Job drawing, mm, ordinate dimensions from the low corner. One solid piece. A direction names the side the tool comes from. Coordinates: 2 decimals unless noted, no trailing zeros. Loops run counter-clockwise (first coordinate to the right, second up) from the corner with the lowest first, then second, coordinate; pieces in that order, holes last. Notation, with made-up numbers: M 31.25,20 L 88.25,20 A22 cw 88.25,48 Z; hole C 43.5,62.25 d1. An arc over 180 degrees is marked long. Answer as a JSON object with one key per item and string values. Group by question number.
1. Drop flat-ended pins along their axis: pin 1 Ø2.5 at (x, z) = (6.5, 5.5) entering from +Y; pin 2 Ø0.7 at (x, z) = (6.5, 5.5) entering from -Y; pin 3 Ø2 at (y, z) = (10.5, 2) entering from +X. Give the stop position or say it passes through.
2. Saw through at D-D on z = 4.25. Write the cut outline in (x, y).
3. Saw through at B-B on z = 7.25. Write the cut outline in (x, y).
4. Saw through at C-C on x = 5.75. Write the cut outline in (y, z).
5. Drill centre lines: L1, parallel to Y at x = 4, z = 3; L2, parallel to Y at x = 6.5, z = 5.75; L3, parallel to X at y = 9, z = 5. Where is each one in solid material? Low to high.
6. Saw through at A-A on x = 4.5. Write the cut outline in (y, z).
7. Mould opens along Y. For the marked faces 1, 2, 3 and 4 say: released by +Y, released by -Y, zero draft, split by the parting line, or undercut.
8. 3-axis set-ups, long thin cutter, end or side, ignore diameter. For the marked faces 5, 6 and 7: which of +Z, -Z, +X, -X, +Y, -Y reach the whole face in a straight line?
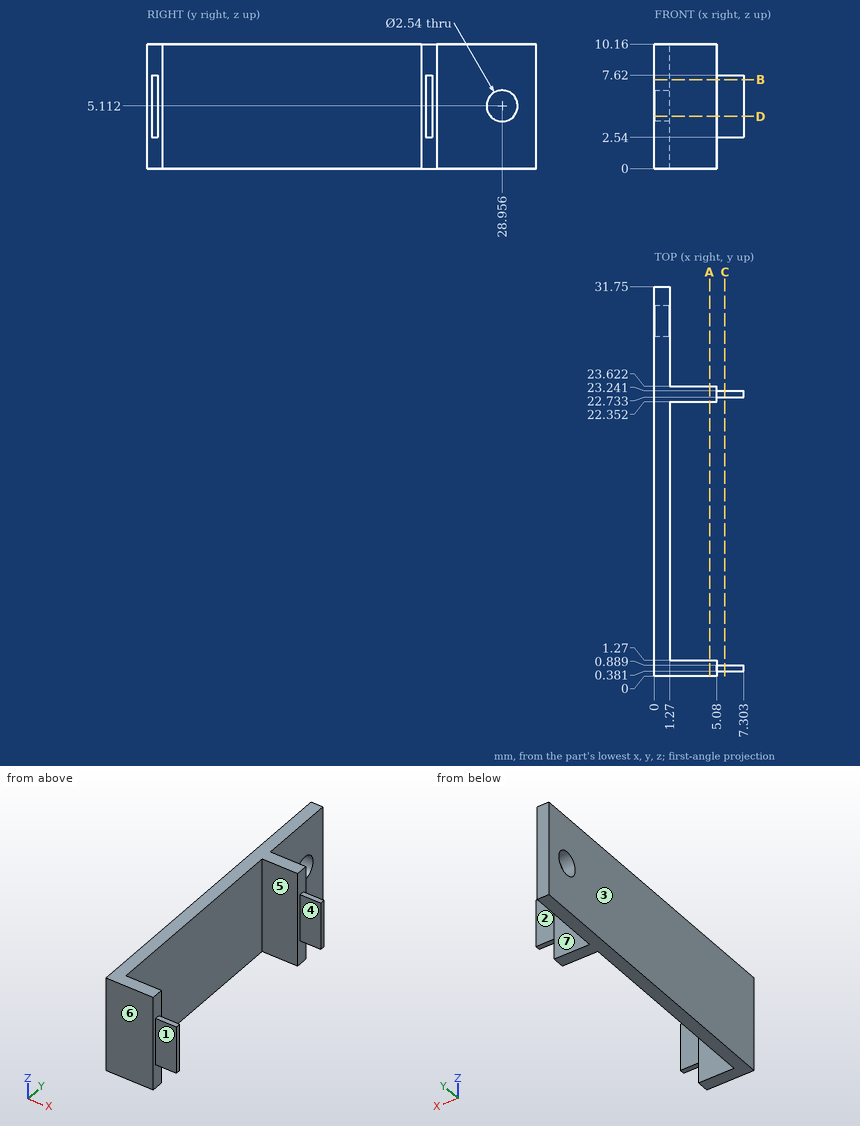
Outcome:
{
 "1": {"pin 1": "stops at y = 23.24", "pin 2": "stops at y = 0.38", "pin 3": "stops at x = 1.27"},
 "2": {"outline": "M 0,0 L 5.08,0 L 5.08,0.38 L 7.3,0.38 L 7.3,0.89 L 5.08,0.89 L 5.08,1.27 L 1.27,1.27 L 1.27,22.35 L 5.08,22.35 L 5.08,22.73 L 7.3,22.73 L 7.3,23.24 L 5.08,23.24 L 5.08,23.62 L 1.27,23.62 L 1.27,28.02 L 0,28.02 Z; M 0,29.89 L 1.27,29.89 L 1.27,31.75 L 0,31.75 Z"},
 "3": {"outline": "M 0,0 L 5.08,0 L 5.08,0.38 L 7.3,0.38 L 7.3,0.89 L 5.08,0.89 L 5.08,1.27 L 1.27,1.27 L 1.27,22.35 L 5.08,22.35 L 5.08,22.73 L 7.3,22.73 L 7.3,23.24 L 5.08,23.24 L 5.08,23.62 L 1.27,23.62 L 1.27,31.75 L 0,31.75 Z"},
 "4": {"outline": "M 0.38,2.54 L 0.89,2.54 L 0.89,7.62 L 0.38,7.62 Z; M 22.73,2.54 L 23.24,2.54 L 23.24,7.62 L 22.73,7.62 Z"},
 "5": {"L1": "y = 0 to 1.27, 22.35 to 23.62", "L2": "y = 0.38 to 0.89, 22.73 to 23.24", "L3": "x = 0 to 1.27"},
 "6": {"outline": "M 0,0 L 1.27,0 L 1.27,10.16 L 0,10.16 Z; M 22.35,0 L 23.62,0 L 23.62,10.16 L 22.35,10.16 Z"},
 "7": {"face 1": "released by -Y", "face 2": "released by +Y", "face 3": "zero draft", "face 4": "undercut"},
 "8": {"face 5": "+Z, -Z, +X", "face 6": "+Z, -Z, +X, -X, -Y", "face 7": "+Z, -Z, +X, +Y"}
}
